CAD build for the part. Positions are in the model's coordinates, mm. Face numbers are marked on the shaded views. Coordinates: 2 decimals unless noted, no trailing zeros. Loops run counter-clockwise (first coordinate to the right, second up) from the corner with the lowest first, then second, coordinate; pieces in that order, holes last.
1) Wall check: line 1 along X through (y, z) = (-19.05, 1) (3 decimals); line 2 along Y through (x, z) = (63.5, 0.7) (3 decimals); line 3 along Y through (x, z) = (63.5, 2) (3 decimals). Give the ranges that are in metal, low to high.
2) Pin check, flat tips, straight feed: pin 1 Ø6 at (y, z) = (-5.5, 10) entering from +X; pin 2 Ø2 at (x, y) = (11, -8.5) entering from +Z; pin 3 Ø1 at (x, z) = (20.5, 9) entering from -Y. Stop position of each tip, or through.
3) Two-plate mould, pull along Z, no slides. Class the marked faces 1, 2, 3 and 4: +Z half, -Z half, draft (parallel to the pull), parting line (faces both ways), or undercut.
4) Saw through at A-A, the plane y = -19.05. Write the cut outline in (x, z) (3 decimals).
5) Saw through at B-B, the plane x = 66. Write the cut outline in (y, z) (3 decimals), and give its area (3 significant figures).
6) Saw through at C-C, the plane z = 1.75. Write the cut outline in (x, y) (3 decimals), and give its area (3 significant figures).
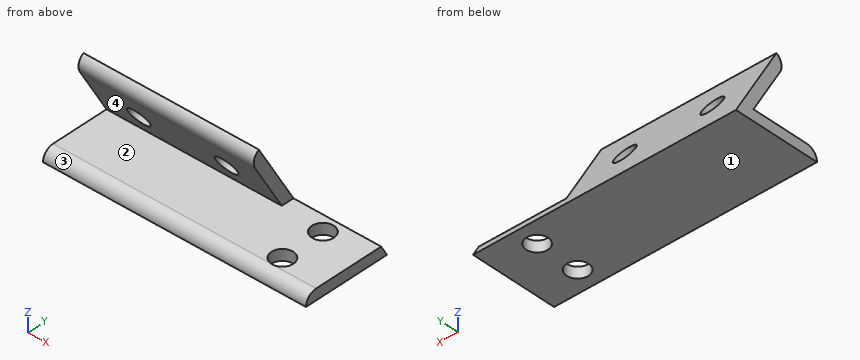
```python
from build123d import *

# Parameters (mm, degrees)
BOSS_EXTRUDE1_DEPTH             = 76.2
CUT_EXTRUDE2_REACH              = 85.279
SKETCH3_W                       = 25.4
SKETCH3_H                       = 25.4
F_1_4_0_25_DIAMETER_HOLE1_D     = 6.35
F_1_4_0_25_DIAMETER_HOLE2_D     = 6.35
F_1_4_0_25_DIAMETER_HOLE2_DEPTH = 3.175


with BuildPart() as part:
    # Sketch1 → Boss-Extrude1 (new body)
    with BuildSketch(Plane(origin=(0, 0, 0), x_dir=(0, 0, -1), z_dir=(1, 0, 0))):
        with BuildLine():
            Line((0, 0), (0, -25.4))
            ThreePointArc((0, -25.4), (-2.24506403, -24.47006403), (-3.175, -22.225))
            Line((-3.175, -22.225), (-3.175, -5.499261314))
            Line((-3.175, -5.499261314), (-17.659914599, -13.862130657))
            ThreePointArc((-17.659914599, -13.862130657), (-20.069165067, -14.179314498), (-21.997045256, -12.7))
            Line((-21.997045256, -12.7), (0, 0))
        make_face()
    extrude(amount=BOSS_EXTRUDE1_DEPTH)

    # Sketch3 → Cut-Extrude2 (cut, up to next)
    with BuildSketch(Plane(origin=(0, 0, 0), x_dir=(1, 0, 0), z_dir=(0, 1, 0)), mode=Mode.PRIVATE) as cut_extrude2_sk1:
        with Locations((63.5, -15.875)):
            Rectangle(SKETCH3_W, SKETCH3_H)
    cut_extrude2_tool1 = extrude(cut_extrude2_sk1.sketch, amount=-CUT_EXTRUDE2_REACH, mode=Mode.PRIVATE) & part.part
    add(cut_extrude2_tool1.solids().sort_by_distance((63.5, 0, 15.875))[0], mode=Mode.SUBTRACT)

    # 1/4 (0.25) Diameter Hole1 (through all)
    with Locations(Plane.XY.offset(3.175)):
        with Locations((63.5, -6.35), (63.5, -19.05)):
            Hole(F_1_4_0_25_DIAMETER_HOLE1_D / 2)

    # 1/4 (0.25) Diameter Hole2
    with Locations(Plane(origin=(0, 0, 0), x_dir=(1, 0, 0), z_dir=(0, 0.8660254037844398, 0.49999999999999806))):
        with Locations((12.7, -12.7), (38.1, -12.7)):
            Hole(F_1_4_0_25_DIAMETER_HOLE2_D / 2, depth=F_1_4_0_25_DIAMETER_HOLE2_DEPTH)


solid = part.part
```
Data:
1. line 1: x = 0 to 60.325, 66.675 to 76.2
1. line 2: y = -25.322 to -22.225, -15.875 to -9.525, -3.175 to -0.404
1. line 3: y = -24.691 to -22.225, -15.875 to -9.525, -3.175 to -1.155
2. pin 1: stops at x = 50.8
2. pin 2: stops at z = 16.45
2. pin 3: stops at y = -9.15
3. face 1: -Z half
3. face 2: undercut
3. face 3: +Z half
3. face 4: undercut
4. outline: (0, 0) - (60.325, 0) - (60.325, 3.175) - (0, 3.175) - close; (66.675, 0) - (76.2, 0) - (76.2, 3.175) - (66.675, 3.175) - close
5. outline: (-25.4, 0) - (-21.007, 0) - (-21.007, 3.175) - (-22.225, 3.175) arc R3.175 ccw to start; (-17.093, 0) - (-8.307, 0) - (-8.307, 3.175) - (-17.093, 3.175) - close; (-4.393, 0) - (0, 0) - (-1.833, 3.175) - (-4.393, 3.175) - close
5. area: 50.7 mm2
6. outline: (0, -24.874) - (76.2, -24.874) - (76.2, -1.01) - (0, -1.01) - close; hole circle Ø6.35 at (63.5, -19.05); hole circle Ø6.35 at (63.5, -6.35)
6. area: 1,760 mm2
